Geometry check sheet. Reference: the model listing, model coordinates, mm. A direction names the side the tool comes from. Coordinates: 2 decimals unless noted, no trailing zeros. Write each loop counter-clockwise with the first axis right and the second up, starting at its lowest first coordinate (ties: lowest second). Pieces come first, ordered by that corner, then holes. Notation, with made-up numbers: M 77.5,-11.75 L 100.5,-11.75 A7 ccw 100.5,-1.75 Z; hole C 15.5,-8 d11. An arc over 180 degrees is marked long. Write item = value, one per line. Start each with the question number.
Autodesk Inventor part; units mm, degrees
ref_plane "Work Plane1" through (29, 0, 0) normal (0, -1, 0) x (1, 0, 0)
ref_plane "YZ Plane" through (0, 0, 0) normal (1, 0, 0) x (0, 1, 0)
ref_plane "XZ Plane" through (0, 0, 0) normal (0, 1, 0) x (-1, 0, 0)
sketch "Sketch1" plane through (0, 0, 0) normal (0, 0, 1) x (1, 0, 0)
  line L0 (0.2, 0) -> (30, 0)
  line L1 (30, 0) -> (30, 2.5)
  line L2 (30, 2.5) -> (14, 2.5)
  line L3 (14, 2.5) -> (13.5091, 2.5)
  line L4 (13.5091, 2.5) -> (0, 2.5)
  line L5 (0, 2.5) -> (0, 4.25)
  line L6 (0, 4.25) -> (-3.5, 4.25)
  line L7 (-3.5, 4.25) -> (-3.5, 1.7321)
  line L8 (-3.5, 1.7321) -> (-0.8, 1.7321)
  line L9 (-0.8, 1.7321) -> (0.2, 0)
  line L10 (-10.2, 0) -> (36.7, 0)
  line L11 (0, -0.85) -> (0, 5.1)
  line L12 (14, 2.5) -> (0, 2.5) construction
  dimension "d1" = 16
  dimension "d2" = 0.4909
  dimension "d3" = 3.5
  dimension "d4" = 2.7
  dimension "d5" = 60
  dimension "d6" = 5
  dimension "d7" = 5
  dimension "d8" = 3.4641
  dimension "d9" = 8.5
  dimension "d26" = 30
revolve "Body" add sketch "Sketch1" angle 360 about axis through (0.2, 0, 0) along (1, 0, 0) contours L9 L11 L4 L3 L2 L1 L0 | L9 L8 L7 L6 L5 L11
sketch "Sketch2" plane through (-3.5, 0, 0) normal (-1, 0, 0) x (0, 0, 1)
  circle A0 centre (0, 0) radius 1.7321
  line L0 (0, -5.95) -> (0, 5.95)
  line L1 (-5.95, 0) -> (5.95, 0)
  line L2 (1.7321, 0) -> (0.866, -1.5)
  line L3 (0.866, -1.5) -> (-0.866, -1.5)
  line L4 (-0.866, -1.5) -> (-1.7321, 0)
  line L5 (-1.7321, 0) -> (-0.866, 1.5)
  line L6 (-0.866, 1.5) -> (0.866, 1.5)
  line L7 (0.866, 1.5) -> (1.7321, 0)
extrude "Slot" add sketch "Sketch2" against normal up to next contours L7 A0 | A0 L2 | L6 L0 A0 | A0 L0 L3 | L0 L6 A0 | A0 L3 L0 | L4 A0 | A0 L5
fillet "Fillet1" radius 0.5 1 edges at (-3.5, -4.25, 0)
thread "Thread"
chamfer "Chamfer1" distance 0.4908 distance2 0.4908 1 edges at (30, -2.5, 0) measured on face at (30, -0.5525, -0.0341)
ref_plane "Work Plane1" through (29, 0, 0) normal (0, -1, 0) x (1, 0, 0)
fillet "Fillet2" radius 0.1 1 edges at (0, -2.5, 0)
equation "\"d1\" = GEL"
equation "\"d3\" = KOH"
equation "\"d4\" = INTI"
equation "\"d6\" = GD"
equation "\"d7\" = BDM"
equation "\"d8\" = 1.1547 * SW"
equation "\"d9\" = KOD"
equation "\"d26\" = NLG"
equation "\"d30\" = R"
equation "\"d17\" = RR"
equation "\"d13\" = GEL"
equation "\"d15\" = -0.5 * SPD + 0.5 * GD"
equation "\"d16\" = GUL"
equation "\"GD\" = NND"
equation "\"NLG\" = 30"
equation "\"GEL\" = 16"
equation "\"KOD\" = 8.5"
equation "\"KOH\" = 3.5"
equation "\"INTI\" = 2.7"
equation "\"GAL\" = 0.61345 * PTC"
equation "\"GUL\" = 0.61345 * PTC"
equation "\"BDM\" = NND"
equation "\"SW\" = 3"
equation "\"RR\" = 0.5"
equation "\"SPD\" = NND - 1.2269 * PTC"
equation "\"R\" = 0.1"
equation "\"TOA\" = 30deg"
equation "\"GD1\" = THREADDIA - 1.2269 * PTC"
equation "\"THREADDIA\" = 5"
equation "\"FAWI\" = 45deg"
equation "\"ANG\" = 120deg"
equation "\"PTC\" = 0.8"
equation "\"NND\" = 5"
equation "\"E0\" = 1.155 * SW"
properties part number "DIN 7984 - M5 x 30" material "Steel, Mild"
Q1. Scan lines: L1, parallel to Y at x = 10.5, z = 2; L2, parallel to Z at x = 25.5, y = 0. Record each from-to range of solid material in increasing order.
Q2. Set-up check for faces 1 (the face through (30, 0, 0)), 2 (the face through (0, 2, 2)), 3 (the face through (-2, -1.5, 0)): record each of +Z, -Z, +X, -X, +Y, -Y from which the full face is reachable in a straight line by a thin tool's end or side.
Q3. Gauge pin test, flat ends, axial feed: pin 1 (1.5 mm diameter, centred on x = 7.5, z = 2.5, fed in from +Y); pin 2 (1.5 mm diameter, centred on x = 19, y = 1, fed in from +Z); pin 3 (0.5 mm diameter, centred on x = -2.5, z = -0.5, fed in from +Y). Record the tip position at first contact, or that the pin passes through.
Q4. Cross-section at A-A on x = 24.5. Enter the section's corners in (y, z).
Q5. Draft check along Y on faces 4 (the face through (-3.5, -2, 0)), 5 (the face through (-2.103, 0.761, 1.293)), 6 (the face through (-1.521, 2.285, -3.584)). Enter one of: pulls with the +Y half, pulls with the -Y half, needs draft (parallel to the pull), parting line crosses it, or undercut.
Values found:
q1.L1 = -1.5 to 1.5
q1.L2 = -2.5 to 2.5
q2.face_1 = +Z, -Z, +X, +Y, -Y
q2.face_2 = +X
q2.face_3 = -X
q3.pin_1 = 1.79
q3.pin_2 = 2.49
q3.pin_3 = 4.24
q4.outline = C 0,0 d5
q5.face_4 = needs draft
q5.face_5 = undercut
q5.face_6 = parting line crosses it
